Here's how the part is built. I have some questions about the finished solid (model axes, mm). A direction names the side the tool comes from. Coordinates: 2 decimals unless noted, no trailing zeros. Write each loop counter-clockwise with the first axis right and the second up, starting at its lowest first coordinate (ties: lowest second). Pieces come first, ordered by that corner, then holes. Notation, with made-up numbers: (56.5, 71.25) -> (113.5, 71.25) arc R17 ccw to (113.5, 83.25) -> close; hole circle Ø11 at (-30.75, 84.5). An arc over 180 degrees is marked (long way). Use a Markdown table: item, result. Add a question column.
Item 1: If we mould it in two halves opening along Y, with no side actions, what happens to faces 4 (the flat face through (-69, 0, 43)), 5 (the flat face through (-9, -31, 101.6)), 6 (the flat face through (-66.713, 17.876, 43.217)), 7 (the cylindrical face through (-25.371, -19.454, 55.268))? For each: pulls with the +Y half, pulls with the -Y half, needs draft (parallel to the pull), parting line crosses it, or undercut.
Item 2: Will these pins go through, and if not, where does the flat tip stop? pin 1 Ø10 at (x, z) = (-57, 32.5) entering from -Y; pin 2 Ø5 at (x, z) = (-15.5, 26) entering from +Y; pin 3 Ø4 at (x, y) = (-11, -14) entering from -Z; pin 4 Ø8 at (x, y) = (-49, 7) entering from -Z.
Item 3: Imagine slicing it at C-C, the plane z = 52. Count the separate pieces of the cut face and the enclosed holes in it, and give its area (3 significant figures).
Item 4: Imagine slicing it at B-B, the plane x = 0. Write out the boundary of the cut face in (y, z), and give its area (3 significant figures).
Item 5: On a 3-axis mill with a long thin cutter (end or side, diameter ignored), from which of +Z, -Z, +X, -X, +Y, -Y can I reach the whole of each face in a straight line? I mean faces 1 (the conical face through (-38.06, 4.94, 90.14)), 2 (the flat face through (0, 0, 7.62)), 3 (the flat face through (-1, 1, 0)). Say none if no direction works.
Item 6: Imagine slicing it at A-A, the plane y = 28. Write out the boundary of the cut face in (x, z), and give its area (3 significant figures).
Item 7: If I drill on line 1 along Y through (x, z) = (0, 69.5); line 2 along X through (y, z) = (8.5, 70); line 3 along X through (y, z) = (13, 45.5), over which ranges is the centre line in solid material (lowest first)? Write a range as from..to.
```python
from build123d import *

# Parameters (mm, degrees)
F0_R     = 38.212329
F1_DEPTH = 101.6
F2_R     = 31.970454
F3_DEPTH = 93.98
F5_ANGLE = 15
F6_R     = 3.81


with BuildPart() as f1:
    # F0 (on Top) → F1 (new body)
    with BuildSketch(Plane.XY):
        Circle(F0_R)
    extrude(amount=F1_DEPTH)

    # F2 (on face) → F3 (cut)
    with BuildSketch(Plane.XY.offset(101.6)):
        Circle(F2_R)
    extrude(amount=-F3_DEPTH, mode=Mode.SUBTRACT)

    # F4 (on Front) → F5 (revolve)
    with BuildSketch(Plane.XZ):
        with BuildLine():
            ThreePointArc((-37.823336, 13.45957), (-65.355852, 48.945968), (-38.440386, 84.90263))
            Line((-38.440386, 84.90263), (-38.323194, 95.239505))
            ThreePointArc((-38.323194, 95.239505), (-75.359479, 49.064441), (-37.929054, 3.208294))
            Line((-37.929054, 3.208294), (-37.823336, 13.45957))
        make_face()
    revolve(axis=Axis((0, 0, 0), (0, 0, -1)), revolution_arc=F5_ANGLE)

    # F6
    f6_edges = [f1.edges().sort_by_distance(p)[0] for p in [
        (-63.130057, 16.915648, 49.147506),
        (-72.792051, 19.504571, 49.209229),
        (-65.357045, 0, 49.147506),
        (-75.359876, 0, 49.209229),
    ]]
    fillet(f6_edges, radius=F6_R)


solid = f1.part
```
Ans:
| question | item | result |
|---|---|---|
| 1 | face 4 | pulls with the -Y half |
| 1 | face 5 | needs draft |
| 1 | face 6 | pulls with the +Y half |
| 1 | face 7 | undercut |
| 2 | pin 1 | stops at y = 0.96 |
| 2 | pin 2 | stops at y = 35.93 |
| 2 | pin 3 | stops at z = 0 |
| 2 | pin 4 | stops at z = 5.47 |
| 3 | separate pieces | 2 |
| 3 | enclosed holes | 1 |
| 3 | area | 1,550 mm^2 |
| 4 | outline | (-38.21, 0) -> (38.21, 0) -> (38.21, 101.6) -> (31.97, 101.6) -> (31.97, 7.62) -> (-31.97, 7.62) -> (-31.97, 101.6) -> (-38.21, 101.6) -> close |
| 4 | area | 1,760 mm^2 |
| 5 | face 1 | none |
| 5 | face 2 | +Z |
| 5 | face 3 | -Z, +X, -X, +Y, -Y |
| 6 | outline | (-26, 0) -> (26, 0) -> (26, 101.6) -> (15.43, 101.6) -> (15.43, 7.62) -> (-15.43, 7.62) -> (-15.43, 101.6) -> (-26, 101.6) -> close |
| 6 | area | 2,380 mm^2 |
| 7 | line 1 | y = -38.21..-31.97, 31.97..38.21 |
| 7 | line 2 | x = -70.03..-58.4, -37.25..-30.82, 30.82..37.25 |
| 7 | line 3 | x = -74.08..-63.86, -35.93..-29.21, 29.21..35.93 |
